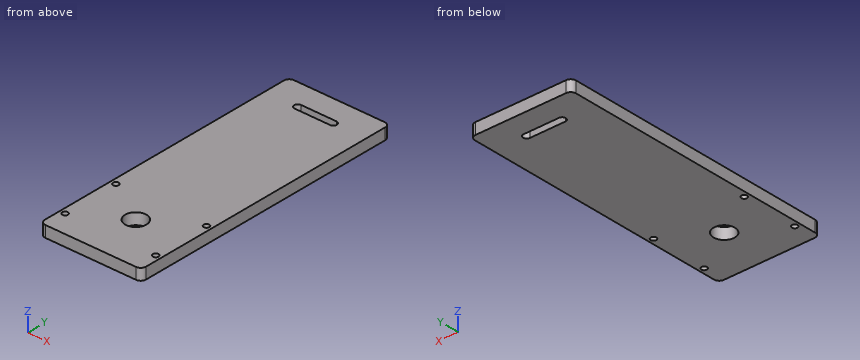
```python
from build123d import *

# Parameters (mm, degrees)
SKETCH1_W           = 57
SKETCH1_H           = 100
SKETCH1_H_2         = 57
SKETCH1_R           = 6
BOSS_EXTRUDE1_DEPTH = 6.35
CUT_EXTRUDE2_DEPTH  = 132.775652152
FILLET1_R           = 3
SKETCH4_R           = 1.6
CUT_EXTRUDE3_DEPTH  = 132.775652152


with BuildPart() as part:
    # Sketch1 → Boss-Extrude1 (new body)
    # profile 1 of 2: a face of its own
    with BuildSketch(Plane.XY):
        with Locations((0, 78.5)):
            Rectangle(SKETCH1_W, SKETCH1_H)
    # profile 2 of 2: a face of its own
    with BuildSketch(Plane.XY):
        Rectangle(SKETCH1_W, SKETCH1_H_2)
        Circle(SKETCH1_R, mode=Mode.SUBTRACT)
    extrude(amount=BOSS_EXTRUDE1_DEPTH)

    # Sketch3 → Cut-Extrude2 (cut, through all)
    with BuildSketch(Plane.XY.offset(6.35)):
        with BuildLine():
            Line((-10, 115.5), (10, 115.5))
            ThreePointArc((10, 115.5), (12, 113.5), (10, 111.5))
            Line((10, 111.5), (-10, 111.5))
            ThreePointArc((-10, 111.5), (-12, 113.5), (-10, 115.5))
        make_face()
    extrude(amount=-CUT_EXTRUDE2_DEPTH, mode=Mode.SUBTRACT)

    # Fillet1
    fillet1_edges = [part.edges().sort_by_distance(p)[0] for p in [
        (-28.5, 128.5, 3.175),
        (28.5, 128.5, 3.175),
        (28.5, -28.5, 3.175),
        (-28.5, -28.5, 3.175),
    ]]
    fillet(fillet1_edges, radius=FILLET1_R)

    # Sketch4 → Cut-Extrude3 (cut, through all)
    with BuildSketch(Plane.XY.offset(6.35)):
        with Locations((25.5, -16)):
            Circle(SKETCH4_R)
        with Locations(Location((-25.5, -16, 0), (0, 0, 180))):
            Circle(SKETCH4_R)
        with Locations(Location((25.5, 16, 0), (0, 0, 180))):
            Circle(SKETCH4_R)
        with Locations((-25.5, 16)):
            Circle(SKETCH4_R)
    extrude(amount=-CUT_EXTRUDE3_DEPTH, mode=Mode.SUBTRACT)


solid = part.part
```
Check sheet for the modelled part. Datum: model origin and axes. Units: mm. Give positions to 0.01 mm unless a question says otherwise; leave off trailing zeros. Loops run counter-clockwise (first coordinate to the right, second up) from the corner with the lowest first, then second, coordinate; pieces in that order, holes last. Notation, with made-up numbers: M 82,48.5 L 140,48.5 A21 ccw 140,82.5 Z; hole C -1.75,7 d8. An arc over 180 degrees is marked long. Answer in a Markdown table with one row per item.
1) Cross-section at C-C (y = 0). Enter the section's corners in (x, z), plus the area to 3 significant figures.
Solutions:
| item | result |
|---|---|
| outline | M -28.5,0 L -6,0 L -6,6.35 L -28.5,6.35 Z; M 6,0 L 28.5,0 L 28.5,6.35 L 6,6.35 Z |
| area | 286 mm^2 |
2) Cross-section at D-D (z = 1.5). Enter the section's corners in (x, y).
Solutions:
| item | result |
|---|---|
| outline | M -28.5,-25.5 A3 ccw -25.5,-28.5 L 25.5,-28.5 A3 ccw 28.5,-25.5 L 28.5,125.5 A3 ccw 25.5,128.5 L -25.5,128.5 A3 ccw -28.5,125.5 Z; hole C -25.5,-16 d3.2; hole C -25.5,16 d3.2; hole M -10,111.5 L 10,111.5 A2 ccw 10,115.5 L -10,115.5 A2 ccw Z; hole C 0,0 d12; hole C 25.5,-16 d3.2; hole C 25.5,16 d3.2 |
3) Depth check by flat-ended pin: pin 1 (3 mm diameter, centred on x = 25.5, y = -16, fed in from -Z). Enter the tip coordinate at first touch or a pass-through.
Solutions:
| item | result |
|---|---|
| pin 1 | passes through |
4) Thickness scan on line 1 (Y direction, x = 25.5, z = 4.5); line 2 (Y direction, x = 0, z = 5); line 3 (Y direction, x = 8.5, z = 0.5). Record the ranges inside material, lowest first.
Solutions:
| item | result |
|---|---|
| line 1 | y = -28.5 to -17.6, -14.4 to 14.4, 17.6 to 128.5 |
| line 2 | y = -28.5 to -6, 6 to 111.5, 115.5 to 128.5 |
| line 3 | y = -28.5 to 111.5, 115.5 to 128.5 |
5) Cross-section at B-B (y = 16). Enter the section's corners in (x, z), plus the area to 3 significant figures.
Solutions:
| item | result |
|---|---|
| outline | M -28.5,0 L -27.1,0 L -27.1,6.35 L -28.5,6.35 Z; M -23.9,0 L 23.9,0 L 23.9,6.35 L -23.9,6.35 Z; M 27.1,0 L 28.5,0 L 28.5,6.35 L 27.1,6.35 Z |
| area | 321 mm^2 |
6) Cross-section at A-A (x = 0). Enter the section's corners in (y, z).
Solutions:
| item | result |
|---|---|
| outline | M -28.5,0 L -6,0 L -6,6.35 L -28.5,6.35 Z; M 6,0 L 111.5,0 L 111.5,6.35 L 6,6.35 Z; M 115.5,0 L 128.5,0 L 128.5,6.35 L 115.5,6.35 Z |
